Source: CAD feature listing. Evaluate the final solid. Frame: model axes, mm. Face numbers are marked on the shaded views. Round coordinates to 2 decimals unless told otherwise and drop trailing zeros. Write each loop counter-clockwise with the first axis right and the second up, starting at its lowest first coordinate (ties: lowest second). Pieces come first, ordered by that corner, then holes.
from build123d import *

# Parameters (mm, degrees)
BOSS_EXTRUDE1_DEPTH = 3
FILLET1_R           = 10
SKETCH2_R           = 1.75
CUT_EXTRUDE1_DEPTH  = 34.970575503
CHAMFER1_SIZE       = 1


with BuildPart() as part:
    # Sketch1 → Boss-Extrude1 (new body)
    with BuildSketch(Plane(origin=(0, 0, 0), x_dir=(1, 0, 0), z_dir=(0, 1, 0))):
        with BuildLine():
            Line((-15, 4.181836343), (-15, 28))
            Line((-15, 28), (15, 28))
            Line((15, 28), (15, 4.181836343))
            ThreePointArc((15, 4.181836343), (18.415475947, -3.063112486), (10.5, -4.287857357))
            ThreePointArc((10.5, -4.287857357), (0, 0), (-10.5, -4.287857357))
            ThreePointArc((-10.5, -4.287857357), (-18.415475947, -3.063112486), (-15, 4.181836343))
        make_face()
    extrude(amount=BOSS_EXTRUDE1_DEPTH)

    # Fillet1
    fillet1_edges = [part.edges().sort_by_distance(p)[0] for p in [
        (-15, 1.5, -4.181836343),
        (15, 1.5, -4.181836343),
    ]]
    fillet(fillet1_edges, radius=FILLET1_R)

    # Sketch2 → Cut-Extrude1 (cut, through all)
    with BuildSketch(Plane(origin=(0, 3, 0), x_dir=(1, 0, 0), z_dir=(0, 1, 0))):
        with Locations(Location((0, 4, 0), (0, 0, 270))):
            Circle(SKETCH2_R)
        with Locations(Location((13.5, -1.630258043, 0), (0, 0, 270))):
            Circle(SKETCH2_R)
        with Locations(Location((-13.5, -1.630258043, 0), (0, 0, 270))):
            Circle(SKETCH2_R)
        with Locations(Location((-10, 11, 0), (0, 0, 270))):
            Circle(SKETCH2_R)
        with Locations(Location((-10, 21, 0), (0, 0, 270))):
            Circle(SKETCH2_R)
        with Locations(Location((10, 21, 0), (0, 0, 270))):
            Circle(SKETCH2_R)
        with Locations(Location((10, 11, 0), (0, 0, 270))):
            Circle(SKETCH2_R)
    extrude(amount=-CUT_EXTRUDE1_DEPTH, mode=Mode.SUBTRACT)

    # Chamfer1
    chamfer1_edges = [part.edges().sort_by_distance(p)[0] for p in [
        (0, 3, -5.75),
        (13.5, 3, -0.119741957),
        (-13.5, 3, -0.119741957),
        (-10, 3, -12.75),
        (-10, 3, -22.75),
        (10, 3, -22.75),
        (10, 3, -12.75),
    ]]
    chamfer(chamfer1_edges, length=CHAMFER1_SIZE)


solid = part.part
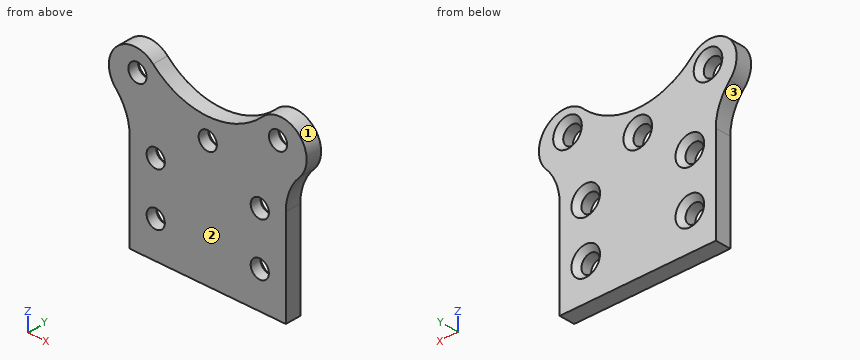
1) Section query D-D on z = -16. Return the cut outline in (x, y), then the cut area to 3 significant figures.
Taken from the geometry:
outline: (-15, 0) - (15, 0) - (15, 3) - (-15, 3) - close
area: 90.0 mm2
2) Material intervals for line 1 (X direction, y = 1.1, z = -21); line 2 (X direction, y = 2.8, z = -20); line 3 (Z direction, x = -11, y = 0.35), sorted ascending.
Taken from the geometry:
line 1: x = -15 to -11.75, -8.25 to 8.25, 11.75 to 15
line 2: x = -15 to -12.35, -7.65 to 7.65, 12.35 to 15
line 3: z = -28 to -22.44, -19.56 to -12.44, -9.56 to 4.72
3) Section query B-B on z = -4. Return the cut outline in (x, y), then the cut area to 3 significant figures.
Taken from the geometry:
outline: (-16.64, 0) - (-1.75, 0) - (-1.75, 2) - (-2.75, 3) - (-16.64, 3) - close; (1.75, 0) - (16.64, 0) - (16.64, 3) - (2.75, 3) - (1.75, 2) - close
area: 88.3 mm2
4) Section query C-C on x = 10. Return the cut outline in (y, z), then the cut area to 3 significant figures.
Taken from the geometry:
outline: (0, -28) - (3, -28) - (3, -23.75) - (2, -22.75) - (0, -22.75) - close; (0, -19.25) - (2, -19.25) - (3, -18.25) - (3, -13.75) - (2, -12.75) - (0, -12.75) - close; (0, -9.25) - (2, -9.25) - (3, -8.25) - (3, 3.82) - (0, 3.82) - close
area: 72.5 mm2
5) Pull-direction query (X, two-part tool) for the marked faces 1, 2 and 3; classes: released by +X, released by -X, zero draft, split by the parting line, or undercut.
Taken from the geometry:
face 1: undercut
face 2: zero draft
face 3: released by -X
6) Contact query for flat-ended pins moving along their axis: P1, Ø4, axis at x = -10, z = -21, coming from the +Y side; P2, Ø12, axis at x = -12.5, z = 0, coming from the -Y side; P3, Ø1.5, axis at y = 1.5, z = -21.5, coming from the -X side; P4, Ø2, axis at x = -10, z = -11, coming from the -Y side. Output: stop coordinate, or through.
Taken from the geometry:
P1: stops at y = 2.25
P2: stops at y = 0
P3: stops at x = -15
P4: passes through
7) Section query A-A on y = 0.55. Return the cut outline in (x, z).
Taken from the geometry:
outline: (-17.67, -2.68) arc R10 cw to (-15, -9.48) - (-15, -28) - (15, -28) - (15, -9.48) arc R10 cw to (17.67, -2.68) arc R5 ccw to (10.5, 4.29) arc R15 cw to (-10.5, 4.29) arc R5 ccw to start; hole circle Ø3.5 at (-13.5, 1.63); hole circle Ø3.5 at (-10, -21); hole circle Ø3.5 at (-10, -11); hole circle Ø3.5 at (0, -4); hole circle Ø3.5 at (10, -21); hole circle Ø3.5 at (10, -11); hole circle Ø3.5 at (13.5, 1.63)
